Read the model definition and answer for the solid it produces. Units are mm, in the model's axes. Face numbers are marked on the shaded views. A direction names the side the tool comes from. Coordinates: 2 decimals unless noted, no trailing zeros. Write each loop counter-clockwise with the first axis right and the second up, starting at its lowest first coordinate (ties: lowest second). Pieces come first, ordered by that corner, then holes. Notation, with made-up numbers: (-20.5, 17) -> (24.5, 17) arc R19 ccw to (24.5, 35) -> close; hole circle Ø10 at (-28, 75.25). An arc over 180 degrees is marked (long way). Use CSV: the item, a comma, the result in double quotes.
from build123d import *

# Parameters (mm, degrees)
F1_DEPTH = 4
F3_D     = 6
F3_DEPTH = 10
F4_R     = 22
F5_DEPTH = 13.5
F6_R     = 18
F7_DEPTH = 8
F8_R     = 10
F9_DEPTH = 25


with BuildPart() as f1:
    # F0 (on Front) → F1 (new body)
    with BuildSketch(Plane.XZ):
        with BuildLine():
            Line((33.42, 96), (-33.42, 96))
            Line((-33.42, 96), (-41.746287, 73.123714))
            ThreePointArc((-41.746287, 73.123714), (-54.305922, 53.409036), (-74.020601, 40.849401))
            Line((-74.020601, 40.849401), (-111, 27.39))
            Line((-111, 27.39), (-111, -27.39))
            Line((-111, -27.39), (-35.447282, -67.227154))
            ThreePointArc((-35.447282, -67.227154), (54.388917, -53.083384), (66.346243, 37.069881))
            Line((66.346243, 37.069881), (33.42, 96))
        make_face()
    extrude(amount=F1_DEPTH)

    # F3
    with Locations(Plane.XZ.offset(4)):
        with Locations((0, 92), (-107, 0), (0, -72), (72, 0)):
            Hole(F3_D / 2, depth=F3_DEPTH)

    # F4 (on face) → F5 (join)
    with BuildSketch(Plane.XZ.offset(4)):
        Circle(F4_R)
    extrude(amount=F5_DEPTH)

    # F6 (on face) → F7 (cut)
    with BuildSketch(Plane.XZ.offset(17.5)):
        Circle(F6_R)
    extrude(amount=-F7_DEPTH, mode=Mode.SUBTRACT)

    # F8 (on face) → F9 (cut)
    with BuildSketch(Plane.XZ.offset(9.5)):
        Circle(F8_R)
    extrude(amount=-F9_DEPTH, mode=Mode.SUBTRACT)


solid = f1.part
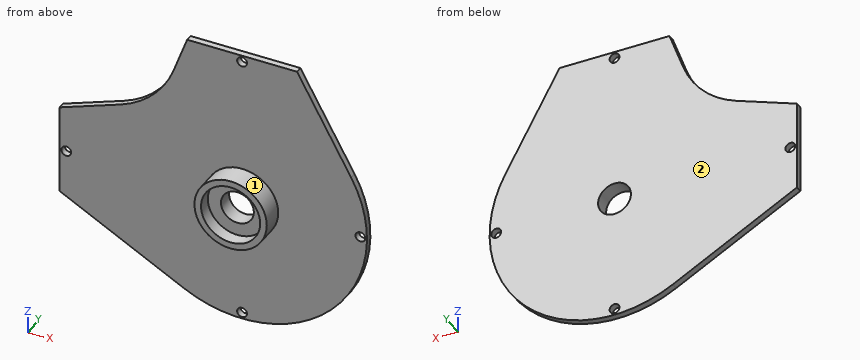
1. A cutting plane is placed at B-B (z = 92). Give the vertices of the cut face in (x, y), and give its area (3 significant figures).
Solutions:
outline,"(-34.88, -4) -> (-3, -4) -> (-3, 0) -> (-34.88, 0) -> close; (3, -4) -> (35.65, -4) -> (35.65, 0) -> (3, 0) -> close"
area,"258 mm^2"
2. Each of these flat-tipped pins is pushed along its axis until it touches: pin 1 Ø3.5 at (x, z) = (0, 92) entering from +Y; pin 2 Ø3 at (x, y) = (-66, -5) entering from +Z; pin 3 Ø1.5 at (x, z) = (-35.5, 55) entering from -Y. Where does it stop, or does it pass through?
Solutions:
pin 1,"passes through"
pin 2,"stops at z = 45.18"
pin 3,"stops at y = -4"
3. A cutting plane is placed at C-C (x = -107). Give the vertices of the cut face in (y, z), and give its area (3 significant figures).
Solutions:
outline,"(-4, -29.5) -> (0, -29.5) -> (0, -3) -> (-4, -3) -> close; (-4, 3) -> (0, 3) -> (0, 28.85) -> (-4, 28.85) -> close"
area,"209 mm^2"
4. Find the intervals of material crossed by line 1 along Z through (x, y) = (0, -1.6); line 2 along Z through (x, y) = (0, -4.5); line 3 along Y through (x, z) = (-39, -63), in increasing order.
Solutions:
line 1,"z = -76 to -75, -69 to -10, 10 to 89, 95 to 96"
line 2,"z = -22 to -10, 10 to 22"
line 3,"y = -4 to 0"
5. A cutting plane is placed at D-D (z = -62.5). Give the vertices of the cut face in (x, y), and give its area (3 significant figures).
Solutions:
outline,"(-44.41, -4) -> (43.24, -4) -> (43.24, 0) -> (-44.41, 0) -> close"
area,"351 mm^2"
6. A cutting plane is placed at A-A (x = 0). Give the vertices of the cut face in (y, z).
Solutions:
outline,"(-17.5, -22) -> (-4, -22) -> (-4, -69) -> (0, -69) -> (0, -10) -> (-9.5, -10) -> (-9.5, -18) -> (-17.5, -18) -> close; (-17.5, 18) -> (-9.5, 18) -> (-9.5, 10) -> (0, 10) -> (0, 89) -> (-4, 89) -> (-4, 22) -> (-17.5, 22) -> close; (-4, -76) -> (0, -76) -> (0, -75) -> (-4, -75) -> close; (-4, 95) -> (0, 95) -> (0, 96) -> (-4, 96) -> close"
7. A tool of negligible diameter and unlimited length cuts with its end or side. For the marked faces 1 and 2, from which of +Z, -Z, +X, -X, +Y, -Y can it reach the whole face along a straight path? Write none if from no direction.
Solutions:
face 1,"-Y"
face 2,"+Z, -Z, +X, -X, +Y"
